```python
from build123d import *

# Parameters (mm, degrees)
F0_R     = 3.175
F1_DEPTH = 19.05


with BuildPart() as f1:
    # F0 (on Front) → F1 (new body)
    with BuildSketch(Plane.XZ):
        with BuildLine():
            Line((0, 127), (0, 0))
            Line((0, 0), (25.4, 0))
            Line((25.4, 0), (25.4, 12.7))
            ThreePointArc((25.4, 12.7), (32.839488, 30.660512), (50.8, 38.1))
            Line((50.8, 38.1), (203.2, 38.1))
            ThreePointArc((203.2, 38.1), (221.160512, 30.660512), (228.6, 12.7))
            Line((228.6, 12.7), (228.6, 0))
            Line((228.6, 0), (254, 0))
            Line((254, 0), (254, 203.2))
            Line((254, 203.2), (0, 127))
        make_face()
        with BuildLine():
            ThreePointArc((222.25, 88.9), (216.670384, 75.429616), (203.2, 69.85))
            Line((203.2, 69.85), (50.8, 69.85))
            ThreePointArc((50.8, 69.85), (37.329616, 75.429616), (31.75, 88.9))
            ThreePointArc((31.75, 88.9), (37.329616, 102.370384), (50.8, 107.95))
            Line((50.8, 107.95), (203.2, 150.7998))
            ThreePointArc((203.2, 150.7998), (216.670384, 145.220184), (222.25, 131.7498))
            Line((222.25, 131.7498), (222.25, 88.9))
        make_face(mode=Mode.SUBTRACT)
        with Locations((127, 154.492649)):
            Circle(F0_R, mode=Mode.SUBTRACT)
    extrude(amount=F1_DEPTH)


solid = f1.part
```
Geometry check sheet. Reference: the model listing, model coordinates, mm. A direction names the side the tool comes from. Give positions to 0.01 mm unless a question says otherwise; leave off trailing zeros. Order: outer loops, then holes, each group sorted by start corner. A loop starts at its lowest first (then second) coordinate and runs counter-clockwise, first axis right, second up. Notation, with made-up numbers: (-33.5, 75.25) - (-1.5, 75.25) arc R18 ccw to (-1.5, 91.25) - close; hole circle Ø4 at (24, 5.25). An arc over 180 degrees is marked (long way). Answer in a Markdown table with one row per item. Add a question column.
Q1. Mould release check, pull along Z, two halves, no side actions. Record for faces 4 (the flat face through (125, 0, 58)), 5 (the flat face through (125.933, -9.392, 129.075)), 6 (the cylindrical face through (220.96, -9.39, 30.86)), 7 (the flat face through (128.778, -9.392, 165.633)): pulls with the +Z half, pulls with the -Z half, needs draft (parallel to the pull), parting line crosses it, or undercut.
Q2. Cross-section at B-B, the plane x = 127. Enter the section's corners in (y, z), then the cut area to 3 significant figures.
Q3. Tool access check on faces 1 (the cylindrical face through (32.64, -9.39, 30.46)), 2 (the flat face through (254, -9, 100)), 3 (the cylindrical face through (216.52, -9.39, 145.37)). Record the directions out of +Z, -Z, +X, -X, +Y, -Y that give a thin tool (end or side, any length) a straight path to the whole face; none if there is none.
Q4. Cross-section at D-D, the plane z = 163. Enter the section's corners in (x, y).
Q5. Cross-section at C-C, the plane y = -3. Enter the section's corners in (x, z) (3 decimals), then the cut area to 3 significant figures.
Q6. Cross-section at A-A, the plane z = 113.5. Enter the section's corners in (x, y).
Q7. Material ranges on probe 1 along X at (y, z) = (-16.5, 88.5); probe 2 along Z at (x, y) = (127, -12.25); probe 3 along X at (y, z) = (-13.25, 12), recorded low to high. Write a range as from..to.
Q8. Gauge pin test, flat ends, axial feed: pin 1 (8 mm diameter, centred on x = 101, y = -7, fed in from +Z); pin 2 (4 mm diameter, centred on x = 112.5, y = -17, fed in from -Z); pin 3 (1 mm diameter, centred on x = 61, y = -16, fed in from +Z). Record the tip position at first contact, or that the pin passes through.
Check values:
| question | item | result |
|---|---|---|
| 1 | face 4 | needs draft |
| 1 | face 5 | undercut |
| 1 | face 6 | pulls with the -Z half |
| 1 | face 7 | pulls with the +Z half |
| 2 | outline | (-19.05, 38.1) - (0, 38.1) - (0, 69.85) - (-19.05, 69.85) - close; (-19.05, 129.37) - (0, 129.37) - (0, 151.32) - (-19.05, 151.32) - close; (-19.05, 157.67) - (0, 157.67) - (0, 165.1) - (-19.05, 165.1) - close |
| 2 | area | 1,160 mm^2 |
| 3 | face 1 | -Z, +Y, -Y |
| 3 | face 2 | +Z, -Z, +X, +Y, -Y |
| 3 | face 3 | +Y, -Y |
| 4 | outline | (120, -19.05) - (254, -19.05) - (254, 0) - (120, 0) - close |
| 5 | outline | (0, 0) - (25.4, 0) - (25.4, 12.7) arc R25.4 cw to (50.8, 38.1) - (203.2, 38.1) arc R25.4 cw to (228.6, 12.7) - (228.6, 0) - (254, 0) - (254, 203.2) - (0, 127) - close; hole (31.75, 88.9) arc R19.05 ccw to (50.8, 69.85) - (203.2, 69.85) arc R19.05 ccw to (222.25, 88.9) - (222.25, 131.75) arc R19.05 ccw to (203.2, 150.8) - (50.8, 107.95) arc R19.05 ccw to start; hole circle Ø6.35 at (127, 154.493) |
| 5 | area | 23,400 mm^2 |
| 6 | outline | (0, -19.05) - (70.54, -19.05) - (70.54, 0) - (0, 0) - close; (222.25, -19.05) - (254, -19.05) - (254, 0) - (222.25, 0) - close |
| 7 | probe 1 | x = 0..31.75, 222.25..254 |
| 7 | probe 2 | z = 38.1..69.85, 129.37..151.32, 157.67..165.1 |
| 7 | probe 3 | x = 0..25.4, 228.6..254 |
| 8 | pin 1 | stops at z = 158.5 |
| 8 | pin 2 | stops at z = 38.1 |
| 8 | pin 3 | stops at z = 145.45 |
